Geometry check sheet. Reference: the model listing, model coordinates, mm. Round coordinates to 2 decimals unless told otherwise and drop trailing zeros. Loops run counter-clockwise (first coordinate to the right, second up) from the corner with the lowest first, then second, coordinate; pieces in that order, holes last.
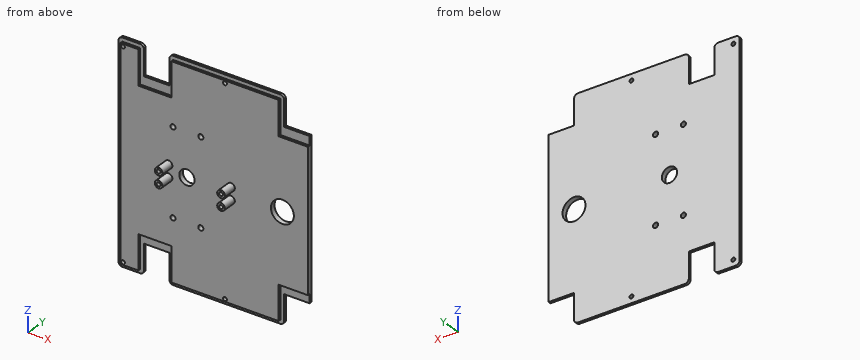
Autodesk Inventor part; units mm, degrees
ref_plane "YZ Plane" through (0, 0, 0) normal (1, 0, 0) x (0, 1, 0)
ref_plane "XZ Plane" through (0, 0, 0) normal (0, 1, 0) x (-1, 0, 0)
ref_plane "XY Plane" through (0, 0, 0) normal (0, 0, 1) x (1, 0, 0)
sketch "Sketch1" plane through (0, 0, 0) normal (0, 1, 0) x (-1, 0, 0)
  line L0 (-66.8277, -81.8282) -> (-43.7605, -81.8282)
  line L1 (-43.7605, -81.8282) -> (-43.7605, -108.8282)
  line L2 (-43.7605, -108.8282) -> (-43.7605, -81.8282)
  line L3 (-43.7605, -108.8282) -> (42.2395, -108.8282)
  line L4 (42.2395, -108.8282) -> (-43.7605, -108.8282)
  line L5 (42.2395, -108.8282) -> (42.2395, -81.8282)
  line L6 (42.2395, -81.8282) -> (66.2395, -81.8282)
  line L7 (66.2395, -81.8282) -> (66.2395, -108.8282)
  line L8 (66.2395, -108.8282) -> (82.1723, -108.8282)
  line L9 (82.1723, -108.8282) -> (82.1723, 57.1718)
  line L10 (82.1723, 57.1718) -> (66.2395, 57.1718)
  line L11 (66.2395, 57.1718) -> (82.1723, 57.1718)
  line L12 (66.2395, 30.1718) -> (42.2395, 30.1718)
  line L13 (42.2395, 30.1718) -> (42.2395, 57.1718)
  line L14 (42.2395, 30.1718) -> (42.2395, 57.1718)
  line L15 (42.2395, 57.1718) -> (-43.7605, 57.1718)
  line L16 (-43.7605, 30.1718) -> (-66.8277, 30.1718)
  line L17 (-66.8277, 30.1718) -> (-43.7605, 30.1718)
  line L18 (-66.8277, 30.1718) -> (-66.8277, -81.8282)
  circle A0 centre (79.2395, -105.8282) radius 1.5
  circle A1 centre (79.2395, -105.8282) radius 1.5
  circle A2 centre (79.2395, 54.1718) radius 1.5
  circle A3 centre (79.2395, 54.1718) radius 1.5
  circle A4 centre (-0.7605, 54.1718) radius 1.5
  circle A5 centre (-0.7605, 54.1718) radius 1.5
  circle A6 centre (-0.7605, -105.8282) radius 1.5
  line L19 (-43.7605, 57.1718) -> (-43.7605, 30.1718)
  line L20 (82.1723, 57.1718) -> (81.1723, 57.1718)
  line L21 (82.1723, 57.1718) -> (82.1723, 56.1718)
  line L22 (66.2395, 57.1718) -> (66.2395, 30.1718)
  line L23 (67.2395, 30.1718) -> (67.2395, 29.1718)
  line L24 (67.2395, 29.1718) -> (42.2395, 29.1718)
  line L25 (42.2395, 57.1718) -> (41.2395, 57.1718)
  line L26 (41.2395, 29.1718) -> (42.2395, 29.1718)
  line L27 (42.2395, 57.1718) -> (42.2395, 56.1718)
  line L28 (-43.7605, 57.1718) -> (-42.7605, 57.1718)
  line L29 (-66.8277, 30.1718) -> (-67.7605, 30.1718)
  line L30 (67.2395, 56.1718) -> (67.2395, 29.1718)
  line L31 (67.2395, 56.1718) -> (81.1723, 56.1718)
  line L32 (81.1723, 56.1718) -> (81.1723, -107.8282)
  line L33 (41.2395, 56.1718) -> (-42.7605, 56.1718)
  line L34 (-42.7605, 56.1718) -> (-42.7605, 29.1718)
  line L35 (41.2395, 56.1718) -> (41.2395, 29.1718)
  line L36 (-65.8277, 29.1718) -> (-65.8277, -80.8282)
  line L37 (-42.7605, 29.1718) -> (-65.8277, 29.1718)
  line L38 (67.2395, -80.8282) -> (42.2395, -80.8282)
  line L39 (41.2395, -80.8282) -> (42.2395, -80.8282)
  line L40 (67.2395, -107.8282) -> (67.2395, -80.8282)
  line L41 (67.2395, -107.8282) -> (81.1723, -107.8282)
  line L42 (41.2395, -107.8282) -> (-42.7605, -107.8282)
  line L43 (-42.7605, -107.8282) -> (-42.7605, -80.8282)
  line L44 (41.2395, -107.8282) -> (41.2395, -80.8282)
  line L45 (-42.7605, -80.8282) -> (-65.8277, -80.8282)
  point P0 (0, 0)
  point P1 (0, 0)
  point P2 (-65.7605, 30.1718)
  dimension "d0" = 1
  dimension "d1" = 1
  dimension "d2" = 1
  dimension "d3" = 1
  dimension "d4" = 1
  dimension "d5" = 1
  dimension "d6" = 1
  dimension "d97" = 1
  dimension "d99" = 84
  dimension "d100" = 25
  dimension "d101" = 27
  dimension "d102" = 1
  dimension "d103" = 147
  dimension "d104" = 1
extrude "Extrusion1" add sketch "Sketch1" along normal blind 2 contours L30 L31 L32 L41 L40 L38 L39 L44 L42 L43 L45 L36 L37 L34 L33 L35 L26 L24 L23
sketch "Sketch4" plane through (0, 2, 0) normal (0, 1, 0) x (1, 0, 0)
  line L0 (65.7605, -36.1718) -> (45.7605, -36.1718)
  line L1 (45.7605, -36.1718) -> (45.7605, -59.1718)
  line L2 (45.7605, -59.1718) -> (-44.2395, -59.1718)
  line L3 (-44.2395, -59.1718) -> (-44.2395, -36.1718)
  line L4 (-44.2395, -59.1718) -> (-44.2395, -36.1718)
  line L5 (-44.2395, -36.1718) -> (-64.2395, -36.1718)
  line L6 (-64.2395, -36.1718) -> (-64.2395, -59.1718)
  line L7 (-64.2395, -59.1718) -> (-84.1723, -59.1718)
  line L8 (-84.1723, -59.1718) -> (-84.1723, 110.8282)
  line L9 (-84.1723, -59.1718) -> (-84.1723, 110.8282)
  line L10 (-84.1723, 110.8282) -> (-64.2395, 110.8282)
  line L11 (-64.2395, 110.8282) -> (-64.2395, 87.8282)
  line L12 (-64.2395, 87.8282) -> (-44.2395, 87.8282)
  line L13 (-44.2395, 87.8282) -> (-44.2395, 110.8282)
  line L14 (-44.2395, 87.8282) -> (-44.2395, 110.8282)
  line L15 (-44.2395, 110.8282) -> (45.7605, 110.8282)
  line L16 (45.7605, 110.8282) -> (45.7605, 87.8282)
  line L17 (45.7605, 87.8282) -> (65.7605, 87.8282)
  line L18 (65.8277, 80.8282) -> (42.7605, 80.8282)
  line L19 (-41.2395, -56.1718) -> (42.7605, -56.1718)
  line L20 (-41.2395, 80.8282) -> (-67.2395, 80.8282)
  line L21 (-81.1723, 107.8282) -> (-81.1723, -56.1718)
  line L22 (42.7605, -56.1718) -> (42.7605, -29.1718)
  line L23 (65.8277, -29.1718) -> (65.8277, 80.8282)
  line L24 (-67.2395, 80.8282) -> (-67.2395, 107.8282)
  line L25 (-67.2395, 107.8282) -> (-81.1723, 107.8282)
  line L26 (-67.2395, -56.1718) -> (-67.2395, -29.1718)
  line L27 (-67.2395, -29.1718) -> (-41.2395, -29.1718)
  line L28 (42.7605, -29.1718) -> (65.8277, -29.1718)
  line L29 (65.7605, 87.8282) -> (65.8277, 87.8282)
  line L30 (65.8277, 87.8282) -> (65.8277, -36.1718)
  line L31 (65.7605, -36.1718) -> (65.8277, -36.1718)
  point P0 (-0.4583, 54.4093)
  point P1 (-0.4583, 54.4093)
  point P2 (65.7605, -59.1718)
  point P3 (65.7605, 110.8282)
  point P4 (67.7605, 110.8282)
  point P5 (67.7605, -59.1718)
  dimension "d40" = 2
  dimension "d53" = 3
  dimension "d54" = 3
  dimension "d55" = 3
  dimension "d56" = 3
  dimension "d57" = 3
  dimension "d58" = 3
  dimension "d59" = 7
  dimension "d60" = 3
  dimension "d61" = 3
  dimension "d62" = 3
  dimension "d63" = 7
extrude "Extrusion2" add sketch "Sketch4" along normal blind 2
sketch "Sketch5" plane through (0, 0, 0) normal (0, -1, 0) x (1, 0, 0)
  circle A0 centre (0.7605, 54.1718) radius 1.5
  circle A1 centre (0.7605, 54.1718) radius 1.5
  circle A2 centre (0.7605, -105.8282) radius 1.5
  circle A3 centre (0.7605, -105.8282) radius 1.5
  circle A4 centre (-79.2395, 54.1718) radius 1.5
  circle A5 centre (-79.2395, 54.1718) radius 1.5
  circle A6 centre (-79.2395, -105.8282) radius 1.5
  circle A7 centre (-79.2395, -105.8282) radius 1.5
  point P0 (0, 0)
extrude "Extrusion3" cut sketch "Sketch5" against normal blind 4
sketch "Sketch8" plane through (0, 4, 0) normal (0, 1, 0) x (1, 0, 0)
  circle A0 centre (-29.0841, 25.8282) radius 6
  line L0 (-29.0841, 25.8282) -> (-43.0841, 25.8282)
  line L1 (-43.0841, 25.8282) -> (-43.0841, 21.3282)
  circle A1 centre (-43.0841, 21.3282) radius 2
  circle A2 centre (-43.0841, 27.2184) radius 2
  line L2 (-29.0841, 25.8282) -> (4.9159, 25.8282)
  line L3 (4.9159, 25.8282) -> (4.9159, 18.2184)
  circle A3 centre (4.9159, 18.2184) radius 2
  circle A4 centre (4.9159, 27.2184) radius 2
  circle A5 centre (-29.0841, 25.8282) radius 35.46
  line L4 (-19.0841, 59.849) -> (-39.0841, 59.849)
  circle A6 centre (-18.1693, 59.5666) radius 2
  line L5 (-29.0841, -9.6318) -> (-29.0841, 40.8935)
  circle A7 centre (-39.9988, 59.5666) radius 2
  circle A8 centre (-18.1693, -7.9102) radius 2
  circle A9 centre (-39.9988, -7.9102) radius 2
  line L6 (-44.2395, -59.1718) -> (45.7605, -59.1718)
  line L7 (-84.1723, 110.8282) -> (-84.1723, -59.1718)
  point P0 (0, 0)
  point P1 (0, 0)
  dimension "d71" = 12
  dimension "d72" = 14
  dimension "d73" = 4.5
  dimension "d74" = 4
  dimension "d75" = 34
  dimension "d76" = 4
  dimension "d77" = 70.92
  dimension "d78" = 20
  dimension "d79" = 4
  dimension "d80" = 85
extrude "Extrusion4" cut sketch "Sketch8" against normal blind 5 contours L2 L5 A0 | A0 L5 L2 | L5 L0 A0 | A0 L0 L5 | A9 A5 | A5 A9 | A8 A5 | A5 A8 | A6 L4 A5 | A5 A6 | L4 A6 A5 | A7 A5 | A5 L4 A7 | L4 A5 A7
sketch "Sketch9" plane through (0, 0, 0) normal (0, -1, 0) x (1, 0, 0)
  arc A0 (7.1961, -19.635) -> (7.1961, -22.635) centre (5.5191, -21.135) ccw
  circle A1 centre (5.5191, -21.135) radius 2.25
  arc A2 (7.1961, -29.135) -> (7.1961, -32.135) centre (5.5191, -30.635) ccw
  circle A3 centre (5.5191, -30.635) radius 2.25
  arc A4 (-45.158, -22.635) -> (-45.158, -19.635) centre (-43.4809, -21.135) ccw
  circle A5 centre (-43.4809, -21.135) radius 2.25
  arc A6 (-45.158, -32.135) -> (-45.158, -29.135) centre (-43.4809, -30.635) ccw
  circle A7 centre (-43.4809, -30.635) radius 2.25
  circle A8 centre (-29.0898, -25.885) radius 6.4
  circle A9 centre (-29.0898, -25.885) radius 5.3776
  circle A10 centre (5.5191, -21.135) radius 3
  circle A11 centre (5.5191, -30.635) radius 3
  circle A12 centre (5.5191, -21.135) radius 1.5
  circle A13 centre (5.5191, -30.635) radius 1.5
  circle A14 centre (-43.4809, -21.135) radius 1.5
  circle A15 centre (-43.4809, -21.135) radius 3
  circle A16 centre (-43.4809, -30.635) radius 1.5
  circle A17 centre (-43.4809, -30.635) radius 3
  point P0 (0, 0)
  point P1 (0, 0)
  point P2 (-18.9809, -25.885)
  dimension "d84" = 6
  dimension "d85" = 6
  dimension "d86" = 3
  dimension "d87" = 3
  dimension "d88" = 3
  dimension "d89" = 6
  dimension "d90" = 3
  dimension "d91" = 6
extrude "Extrusion5" add sketch "Sketch9" along normal blind 11 contours A1 A0 | A3 A2 | A5 A4 | A7 A6 | A10 | A11 | A15 | A17
fillet "Fillet1" radius 3 8 edges at (-84.1723, 3, 59.1718) (-64.2395, 3, 59.1718) (-44.2395, 3, 59.1718) (45.7605, 3, 59.1718) (-84.1723, 3, -110.8282) (-64.2395, 3, -110.8282) (-44.2395, 3, -110.8282) (45.7605, 3, -110.8282)
sketch "Sketch13" plane through (0, 4, 0) normal (0, 1, 0) x (1, 0, 0)
  circle A0 centre (45.8277, 25.8282) radius 9
  line L0 (65.8277, -36.1718) -> (65.8277, 87.8282)
  point P0 (0, 0)
  dimension "d117" = 18
  dimension "d118" = 20
extrude "Extrusion7" cut sketch "Sketch13" against normal blind 10
properties part number "vrch1"
1) Sectioned sample at C-C, the plane x = 13. Record the cut outline in (y, z).
Report:
outline: (0, -107.83) - (2, -107.83) - (2, -110.83) - (4, -110.83) - (4, 59.17) - (2, 59.17) - (2, 56.17) - (0, 56.17) - close
2) Scan lines: line 1 along Z through (x, y) = (-40, 3); line 2 along X through (y, z) = (0.5, -97); line 3 along Y through (x, z) = (-70.5, 30.5). Record each from-to range of solid material in increasing order.
Report:
line 1: z = -110.83 to -61.57, -57.57 to 5.91, 9.91 to 59.17
line 2: x = -81.17 to -67.24, -41.24 to 42.76
line 3: y = 0 to 4
3) Sectioned sample at D-D, the plane z = -83. Record the cut outline in (x, y).
Report:
outline: (-84.17, 2) - (-81.17, 2) - (-81.17, 0) - (-67.24, 0) - (-67.24, 2) - (-41.24, 2) - (-41.24, 0) - (42.76, 0) - (42.76, 2) - (65.83, 2) - (65.83, 4) - (-84.17, 4) - close
4) Gauge pin test, flat ends, axial feed: pin 1 (1 mm diameter, centred on y = 1, z = -56, fed in from -X); pin 2 (5 mm diameter, centred on x = 48, y = -1, fed in from +Z); pin 3 (2 mm diameter, centred on y = 0.5, z = -96, fed in from +X); pin 4 (5 mm diameter, centred on x = 5.52, z = -21.14, fed in from -Y). Record the tip position at first contact, or that the pin passes through.
Report:
pin 1: stops at x = -81.17
pin 2: stops at z = 29.17
pin 3: stops at x = 42.76
pin 4: stops at y = -11
5) Sectioned sample at B-B, the plane y = -5. Record the cut outline in (x, z) (3 decimals), then the cut area to 3 significant figures.
Report:
outline: circle Ø6 at (-43.481, -30.635); circle Ø6 at (-43.481, -21.135); circle Ø6 at (5.519, -30.635); circle Ø6 at (5.519, -21.135); hole circle Ø3 at (-43.481, -30.635); hole circle Ø3 at (-43.481, -21.135); hole circle Ø3 at (5.519, -30.635); hole circle Ø3 at (5.519, -21.135)
area: 84.8 mm2
6) Sectioned sample at A-A, the plane z = 42. Record the cut outline in (x, y).
Report:
outline: (-84.17, 2) - (-81.17, 2) - (-81.17, 0) - (-67.24, 0) - (-67.24, 2) - (-64.24, 2) - (-64.24, 4) - (-84.17, 4) - close; (-44.24, 2) - (-41.24, 2) - (-41.24, 0) - (42.76, 0) - (42.76, 2) - (45.76, 2) - (45.76, 4) - (-44.24, 4) - close
